Work out the finished part from the listing and answer in its coordinate system (mm). Give positions to 0.01 mm unless a question says otherwise; leave off trailing zeros. Loops run counter-clockwise (first coordinate to the right, second up) from the corner with the lowest first, then second, coordinate; pieces in that order, holes last. Notation, with made-up numbers: (6.5, 3) - (48.5, 3) arc R9 ccw to (48.5, 19) - close; hole circle Ø8 at (-14.5, 33.5). An arc over 180 degrees is marked (long way). One line per question, with ' | ' between items. Start each with the question number.
1. For a pull along X with two mould halves and no side action, classify faces 1 (the face through (-3, 4, -3)), 2 (the face through (-188, 8, 119)) as released by +X, released by -X, zero draft, split by the parting line, or undercut.
2. Each of these flat-tipped pins is pushed along its axis until it touches: pin 1 (3 mm diameter, centred on x = -187.5, y = 7, fed in from -Z); pin 2 (3 mm diameter, centred on x = -18.5, y = 7, fed in from +Z); pin 3 (2 mm diameter, centred on x = 63, y = 6, fed in from +Z); pin 4 (1.2 mm diameter, centred on y = 6.5, z = 119, fed in from +X). Where does it stop, or does it pass through?
3. Find the intervals of material crossed by line 1 (Z direction, x = 92.5, y = 5.25); line 2 (X direction, y = 7.75, z = -18); line 3 (X direction, y = 0.5, z = 139), in increasing order.
4. Section B-B (z = -144.5) is taken. Determine the outline of the cut face in (x, y).
5. Section C-C (x = -173) is taken. Determine the outline of the cut face in (y, z).
6. Section D-D (x = 137.5) is taken. Determine the outline of the cut face in (y, z).
7. Section A-A (y = 5.5) is taken. Give the number of separate pieces and of enclosed holes in the cut face, plus the area to 3 significant figures.
from build123d import *

# Parameters (mm, degrees)
SKETCH1_W            = 500
SKETCH1_H            = 370
PANEL_BASE_DEPTH     = 4
SKETCH2_W            = 65
SKETCH2_H            = 100
SOLAR_ARRAY_DEPTH    = 4
LPATTERN1_COUNT      = 4
LPATTERN1_PITCH      = 124
LPATTERN1_COUNT_DIR2 = 3
LPATTERN1_PITCH_DIR2 = 115
SKETCH3_R            = 1.5
POSITIVE_WIRE_DEPTH  = 30
SKETCH4_R            = 1.5
NEGATIVE_WIRE_DEPTH  = 30


with BuildPart() as part:
    # Sketch1 → panel_base (new body)
    with BuildSketch(Plane(origin=(0, 0, 0), x_dir=(1, 0, 0), z_dir=(0, 1, 0))):
        Rectangle(SKETCH1_W, SKETCH1_H)
    extrude(amount=PANEL_BASE_DEPTH)

    # Sketch2 → solar_array (add)
    with BuildSketch(Plane(origin=(0, 4, 0), x_dir=(1, 0, 0), z_dir=(0, 1, 0))):
        with Locations((-187.5, 110)):
            Rectangle(SKETCH2_W, SKETCH2_H)
    solar_array = extrude(amount=SOLAR_ARRAY_DEPTH)

    # LPattern1: solar_array 4 × 3
    with Locations(*[(i * LPATTERN1_PITCH, 0, j * LPATTERN1_PITCH_DIR2) for i in range(LPATTERN1_COUNT) for j in range(LPATTERN1_COUNT_DIR2) if (i, j) != (0, 0)]):
        add(solar_array)

    # Sketch3 → positive_wire (add)
    with BuildSketch(Plane.ZY.offset(250)):
        with Locations(Location((-8, 1.930294272, 0), (0, 0, 180))):
            Circle(SKETCH3_R)
    extrude(amount=POSITIVE_WIRE_DEPTH)

    # Sketch4 → negative_wire (add)
    with BuildSketch(Plane.ZY.offset(250)):
        with Locations(Location((8, 2.146306887, 0), (0, 0, 180))):
            Circle(SKETCH4_R)
    extrude(amount=NEGATIVE_WIRE_DEPTH)


solid = part.part
Conclusion:
1) face 1: undercut | face 2: zero draft
2) pin 1: z = -160 | pin 2: through | pin 3: z = 170 | pin 4: x = 217
3) line 1: -160 to -60, -45 to 55, 70 to 170 | line 2: -220 to -155, -96 to -31, 28 to 93, 152 to 217 | line 3: -250 to 250
4) outline: (-250, 0) - (250, 0) - (250, 4) - (217, 4) - (217, 8) - (152, 8) - (152, 4) - (93, 4) - (93, 8) - (28, 8) - (28, 4) - (-31, 4) - (-31, 8) - (-96, 8) - (-96, 4) - (-155, 4) - (-155, 8) - (-220, 8) - (-220, 4) - (-250, 4) - close
5) outline: (0, -185) - (4, -185) - (4, -160) - (8, -160) - (8, -60) - (4, -60) - (4, -45) - (8, -45) - (8, 55) - (4, 55) - (4, 70) - (8, 70) - (8, 170) - (4, 170) - (4, 185) - (0, 185) - close
6) outline: (0, -185) - (4, -185) - (4, 185) - (0, 185) - close
7) separate pieces: 12 | enclosed holes: 0 | area: 78,000 mm²
